Here's how the part is built. I have some questions about the finished solid (model axes, mm). A direction names the side the tool comes from. Give positions to 0.01 mm unless a question says otherwise; leave off trailing zeros. Write each loop counter-clockwise with the first axis right and the second up, starting at its lowest first coordinate (ties: lowest second). Pieces come first, ordered by that corner, then holes. Notation, with made-up numbers: (-21.5, 12.25) -> (34.5, 12.25) arc R17 cw to (34.5, 45.25) -> close; hole circle Ø1 at (20, 3.5). An arc over 180 degrees is marked (long way). Put each result on its own line as item: value. Start each with the question number.
from build123d import *

# Parameters (mm, degrees)
F1_DEPTH = 70
F3_DEPTH = 33
F4_R     = 12


with BuildPart() as f1:
    # F0 (on Top) → F1 (new body)
    with BuildSketch(Plane.XY):
        Polygon((14, -16), (16, -16), (16, 16), (-16, 16), (-16, -16), (-14, -16), (-14, 14), (14, 14), align=None)
    extrude(amount=F1_DEPTH)

    # F2 (on face) → F3 (cut)
    with BuildSketch(Plane(origin=(-16, 0, 0), x_dir=(0, -1, 0), z_dir=(-1, 0, 0))):
        Polygon((16, 70), (-16, 70), (16, 0), align=None)
    extrude(amount=-F3_DEPTH, mode=Mode.SUBTRACT)

    # F4
    f4_edges = [f1.edges().sort_by_distance(p)[0] for p in [
        (16, 16, 35),
        (-16, 16, 35),
        (-14, 14, 32.8125),
        (14, 14, 32.8125),
    ]]
    fillet(f4_edges, radius=F4_R)


solid = f1.part
1) Thinking about a two-plate mould opening in X: for faces 1 (the cylindrical face through (12.58, 12.39, 27.71)), 2 (the cylindrical face through (-12.39, 12.58, 27.71)), 3 (the flat face through (-14, -3, 11)), which applies, released by +X, released by -X, zero draft, split by the parting line, or undercut?
2) I want a section at C-C, the plane x = -0.5. Write out the boundary of the cut face in (y, z) (3 decimals).
3) I need wall thicknesses on probe 1 along X at (y, z) = (1, 5.5); probe 2 along X at (y, z) = (3.5, 11); probe 3 along Y at (x, z) = (-12, 39). Which ranges of each line are inside material? Lowest first, please.
4) I want a section at B-B, the plane z = 62. Write out the boundary of the cut face in (x, y), and give its area (3 significant figures).
5) I'm going to push flat-ended pins straight in: pin 1 Ø2 at (x, z) = (-1, 34.5) entering from -Y; pin 2 Ø4 at (x, z) = (5, 23.5) entering from -Y; pin 3 Ø10 at (y, z) = (4.5, 55) entering from -X. Where does each tip first touch, or does it pass through?
6) I want a section at A-A, the plane y = 7. Write out the boundary of the cut face in (x, z), and give its area (3 significant figures).
7) I want a section at D-D, the plane y = -10. Write out the boundary of the cut face in (x, z) (3 decimals), and give its area (3 significant figures).
8) Which directions (+Z, -Z, +X, -X, +Y, -Y) give clear straight access to the entire face, cutting with the end or side of a thin tool? Please do faces 4 (the flat face through (0, 16, 35)), 5 (the cylindrical face through (-10.58, 10.39, 25.98)).
Established:
1. face 1: released by +X
1. face 2: released by -X
1. face 3: undercut
2. outline: (14, 0) -> (16, 0) -> (16, 70) -> (14, 65.625) -> close
3. probe 1: x = -16 to -14, 14 to 16
3. probe 2: x = -16 to -13.91, 13.91 to 16
3. probe 3: y = 8.63 to 12.94
4. outline: (-12.63, 12.34) -> (-8.08, 12.34) arc R12 cw to (-2, 14) -> (2, 14) arc R12 cw to (8.08, 12.34) -> (12.63, 12.34) arc R12 ccw to (4, 16) -> (-4, 16) arc R12 ccw to start
4. area: 52.5 mm2
5. pin 1: stops at y = 14
5. pin 2: stops at y = 12.91
5. pin 3: stops at x = -15.56
6. outline: (-15.62, 0) -> (-12.91, 0) -> (-12.91, 50.31) -> (-15.62, 50.31) -> close; (12.91, 0) -> (15.62, 0) -> (15.62, 50.31) -> (12.91, 50.31) -> close
6. area: 273 mm2
7. outline: (-16, 0) -> (-14, 0) -> (-14, 13.125) -> (-16, 13.125) -> close; (14, 0) -> (16, 0) -> (16, 13.125) -> (14, 13.125) -> close
7. area: 52.5 mm2
8. face 4: +Z, -Z, +X, -X, +Y
8. face 5: +Z, -Z, -Y
